The listing builds one solid part. Answer for the finished solid, in the listing's coordinates (mm). Round coordinates to 2 decimals unless told otherwise and drop trailing zeros. Write each loop counter-clockwise with the first axis right and the second up, starting at its lowest first coordinate (ties: lowest second). Pieces come first, ordered by that corner, then holes.
from build123d import *

# Parameters (mm, degrees)
SKETCH1_W               = 130
SKETCH1_H               = 120
BOSS_EXTRUDE1_DEPTH     = 3
CUT_EXTRUDE1_START      = -4
SKETCH2_W               = 20
SKETCH2_H               = 95
CUT_EXTRUDE1_DEPTH      = 5
CUT_EXTRUDE2_START      = -4
SKETCH3_R               = 6
CUT_EXTRUDE2_DEPTH      = 5
SKETCH4_W               = 130
SKETCH4_H               = 3
BOSS_EXTRUDE2_DEPTH     = 140
SKETCH5_W               = 70
SKETCH5_H               = 6
CUT_EXTRUDE3_DEPTH      = 1
CUT_EXTRUDE3_DEPTH_BACK = 4
FILLET1_R               = 10


with BuildPart() as part:
    # Sketch1 → Boss-Extrude1 (new body)
    with BuildSketch(Plane(origin=(0, 0, 0), x_dir=(1, 0, 0), z_dir=(0, 1, 0))):
        Rectangle(SKETCH1_W, SKETCH1_H)
    extrude(amount=BOSS_EXTRUDE1_DEPTH)

    # Sketch2 → Cut-Extrude1 (cut)
    with BuildSketch(Plane(origin=(0, 3, 0), x_dir=(1, 0, 0), z_dir=(0, 1, 0)).offset(CUT_EXTRUDE1_START)):
        with Locations((-16.25, 0)):
            Rectangle(SKETCH2_W, SKETCH2_H)
    cut_extrude1 = extrude(amount=CUT_EXTRUDE1_DEPTH, mode=Mode.SUBTRACT)

    # Mirror1: Cut-Extrude1 across plane
    add(cut_extrude1.mirror(Plane(origin=(0, 0, 0), x_dir=(0, 0, 1), z_dir=(1, 0, 0))), mode=Mode.SUBTRACT)

    # Sketch3 → Cut-Extrude2 (cut)
    with BuildSketch(Plane(origin=(0, 3, 0), x_dir=(1, 0, 0), z_dir=(0, 1, 0)).offset(CUT_EXTRUDE2_START)):
        with Locations((44.5, 0)):
            Circle(SKETCH3_R)
    cut_extrude2 = extrude(amount=CUT_EXTRUDE2_DEPTH, mode=Mode.SUBTRACT)

    # Mirror2: Cut-Extrude2 across plane
    add(cut_extrude2.mirror(Plane(origin=(0, 0, 0), x_dir=(0, 0, 1), z_dir=(1, 0, 0))), mode=Mode.SUBTRACT)

    # Sketch4 → Boss-Extrude2 (add)
    with BuildSketch(Plane.XY.offset(60)):
        with Locations((0, 1.5)):
            Rectangle(SKETCH4_W, SKETCH4_H)
    extrude(amount=BOSS_EXTRUDE2_DEPTH)

    # Sketch5 → Cut-Extrude3 (cut, two sides)
    with BuildSketch(Plane(origin=(0, 3, 0), x_dir=(1, 0, 0), z_dir=(0, 1, 0))) as cut_extrude3_sk:
        with Locations((0, -75)):
            Rectangle(SKETCH5_W, SKETCH5_H)
        with Locations((0, -191)):
            Rectangle(SKETCH5_W, SKETCH5_H)
    extrude(amount=CUT_EXTRUDE3_DEPTH, mode=Mode.SUBTRACT)
    extrude(cut_extrude3_sk.sketch, amount=-CUT_EXTRUDE3_DEPTH_BACK, mode=Mode.SUBTRACT)

    # Fillet1
    fillet1_edges = [part.edges().sort_by_distance(p)[0] for p in [
        (-65, 1.5, 200),
        (65, 1.5, 200),
        (-65, 1.5, -60),
        (65, 1.5, -60),
    ]]
    fillet(fillet1_edges, radius=FILLET1_R)


solid = part.part
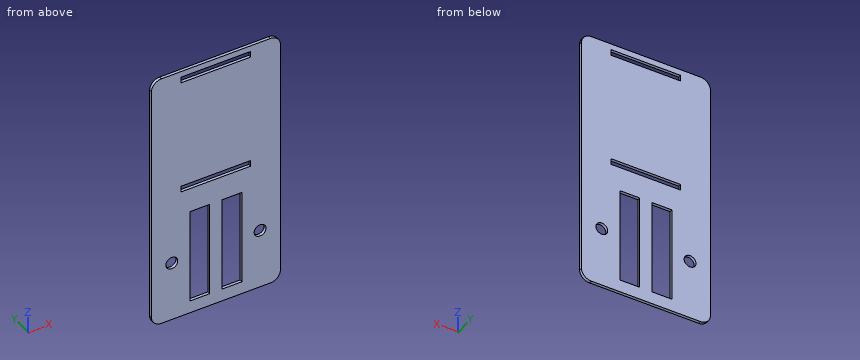
1. Section B-B on x = 44.5 is taken. Determine the outline of the cut face in (y, z), plus the area to 3 significant figures.
Geometry says:
outline: (0, -60) - (3, -60) - (3, -6) - (0, -6) - close; (0, 6) - (3, 6) - (3, 200) - (0, 200) - close
area: 744 mm2
2. Section D-D on y = 1 is taken. Determine the outline of the cut face in (x, z).
Geometry says:
outline: (-65, -50) arc R10 ccw to (-55, -60) - (55, -60) arc R10 ccw to (65, -50) - (65, 190) arc R10 ccw to (55, 200) - (-55, 200) arc R10 ccw to (-65, 190) - close; hole circle Ø12 at (-44.5, 0); hole (-35, 72) - (35, 72) - (35, 78) - (-35, 78) - close; hole (-35, 188) - (35, 188) - (35, 194) - (-35, 194) - close; hole (-26.25, -47.5) - (-6.25, -47.5) - (-6.25, 47.5) - (-26.25, 47.5) - close; hole (6.25, -47.5) - (26.25, -47.5) - (26.25, 47.5) - (6.25, 47.5) - close; hole circle Ø12 at (44.5, 0)
3. Section A-A on z = -22.5 is taken. Determine the outline of the cut face in (x, y), plus the area to 3 significant figures.
Geometry says:
outline: (-65, 0) - (-26.25, 0) - (-26.25, 3) - (-65, 3) - close; (-6.25, 0) - (6.25, 0) - (6.25, 3) - (-6.25, 3) - close; (26.25, 0) - (65, 0) - (65, 3) - (26.25, 3) - close
area: 270 mm2
4. Straight lines are drawn through the part: line 1 along Z through (x, y) = (-18.5, 2.65); line 2 along Z through (x, y) = (30, 2.85); line 3 along X through (y, z) = (1.75, 29.5). For each, find the intervals that lie inside material, in ascending order.
Geometry says:
line 1: z = -60 to -47.5, 47.5 to 72, 78 to 188, 194 to 200
line 2: z = -60 to 72, 78 to 188, 194 to 200
line 3: x = -65 to -26.25, -6.25 to 6.25, 26.25 to 65
5. Given pin 1 (6 mm diameter, centred on x = 11, z = 60.5, fed in from -Y); pin 2 (1.5 mm diameter, centred on y = 2, z = 191.5, fed in from +X), each flat-ended and moving along its own axis, determine where each tip first touches the part or whether it passes through.
Geometry says:
pin 1: stops at y = 0
pin 2: stops at x = 64.97
6. Section C-C on x = 15 is taken. Determine the outline of the cut face in (y, z), plus the area to 3 significant figures.
Geometry says:
outline: (0, -60) - (3, -60) - (3, -47.5) - (0, -47.5) - close; (0, 47.5) - (3, 47.5) - (3, 72) - (0, 72) - close; (0, 78) - (3, 78) - (3, 188) - (0, 188) - close; (0, 194) - (3, 194) - (3, 200) - (0, 200) - close
area: 459 mm2
